Build history of the part. All positions in model axes, mm. Round coordinates to 2 decimals unless told otherwise and drop trailing zeros. Write each loop counter-clockwise with the first axis right and the second up, starting at its lowest first coordinate (ties: lowest second). Pieces come first, ordered by that corner, then holes. Notation, with made-up numbers: (-18, 64) - (-13, 64) arc R14 ccw to (-13, 81) - close; hole circle Ø2 at (69, 71). An arc over 180 degrees is marked (long way). Write each question's results on one line, items separated by ' | '.
Autodesk Inventor part; units mm, degrees
ref_plane "Work Plane1" through (-4668.2945, 0, 0) normal (0, 0, 1) x (1, 0, 0)
ref_plane "YZ Plane" through (0, 0, 0) normal (1, 0, 0) x (0, 1, 0)
ref_plane "XZ Plane" through (0, 0, 0) normal (0, 1, 0) x (-1, 0, 0)
ref_plane "Work Plane1" through (-4668.2945, 0, 0) normal (0, 0, 1) x (1, 0, 0)
sketch "Sketch1" plane through (-4668.2945, 0, 0) normal (0, 0, 1) x (1, 0, 0)
  line L0 (0, 19.05) -> (466.725, 19.05)
  line L1 (466.725, 0) -> (466.725, 19.05)
  line L2 (0, 0) -> (0, 19.05)
  line L3 (0, -340.481) -> (0, -321.431)
  line L4 (466.725, -340.481) -> (0, -340.481)
  line L5 (466.725, -340.481) -> (0, -340.481)
  line L6 (466.725, -340.481) -> (466.725, -321.431)
  line L7 (0, -321.431) -> (466.725, -321.431) construction
  line L8 (0, -340.481) -> (0, -321.431)
  line L9 (466.725, 19.05) -> (0, 19.05)
  line L10 (0, 19.05) -> (0, -340.481) construction
  line L11 (466.725, -340.481) -> (466.725, 19.05) construction
  line L12 (147.3639, -408.7465) -> (46.3111, -408.7465) construction
  line L13 (466.725, -340.481) -> (466.725, -408.7465) construction
  line L14 (466.725, -408.7465) -> (147.3639, -408.7465) construction
  line L15 (46.3111, -408.7465) -> (0, -408.7465)
  line L16 (0, -408.7465) -> (0, -340.481) construction
  line L17 (466.725, -408.7465) -> (466.725, -434.1465)
  line L18 (466.725, -434.1465) -> (0, -434.1465)
  line L19 (0, -434.1465) -> (0, -408.7465)
  line L20 (400.05, 19.05) -> (400.05, 0)
  line L21 (400.05, -321.431) -> (400.05, -340.481)
  line L22 (400.05, 0) -> (400.05, -321.431)
  line L23 (400.05, -340.481) -> (400.05, -434.1465)
  line L24 (101.6, 19.05) -> (101.6, 0)
  line L25 (101.6, -321.431) -> (101.6, -340.481)
  line L26 (101.6, 0) -> (101.6, -321.431)
  line L27 (101.6, -340.481) -> (101.6, -434.1465)
  point P0 (4668.2945, 0)
  point P1 (50.8, 19.05)
  point P2 (50.8, -321.431)
  point P3 (50.8, -340.481)
  point P4 (50.8, -434.1465)
  dimension "d7" = 25.4
extrude "Extrusion1" add sketch "Sketch1" along normal blind 19.05
sketch "Sketch2" plane through (-4668.2945, 0, 0) normal (0, 0, -1) x (-1, 0, 0)
  line L0 (-232.5687, -355.978) -> (-232.5688, 34.547)
  line L1 (-141.2875, -408.7465) -> (-141.2875, 124.6535)
  circle A0 centre (-186.9249, -370.6465) radius 15.875
  line L2 (-232.5687, -370.6465) -> (-141.2875, -370.6465) construction
  line L3 (0, -408.7465) -> (-466.725, -408.7465)
  point P0 (-4668.2945, 0)
  dimension "d2" = 31.75
  dimension "d3" = 45.6438
  dimension "d4" = 38.1
extrude "Extrusion2" cut sketch "Sketch2" against normal up to next
sketch "Sketch3" plane through (-4668.2945, 0, 0) normal (0, 0, -1) x (-1, 0, 0)
  circle A0 centre (-186.9249, -370.6465) radius 15.875
  arc A1 (-207.9625, -430.5603) -> (-155.5881, -425.8756) centre (-186.9249, -370.6465) ccw
  line L0 (-101.6, -434.1465) -> (-400.05, -434.1465)
  line L1 (0, -340.481) -> (-157.1625, -426.7397)
  line L2 (-466.725, -340.481) -> (-207.9625, -430.5603)
  line L3 (-466.725, -434.1465) -> (-466.725, -340.481)
  line L4 (-466.725, -434.1465) -> (-466.725, 19.05)
  line L5 (-101.6, -434.1465) -> (-400.05, -434.1465)
  line L6 (0, -434.1465) -> (0, -340.481)
  line L7 (0, 19.05) -> (0, -434.1465)
  arc A2 (-155.5881, -425.8756) -> (-207.9625, -430.5603) centre (-186.9249, -370.6465) ccw construction
  line L8 (-101.6, 19.05) -> (-101.6, -434.1465)
  line L9 (-101.6, -396.2442) -> (-101.6, -434.1465)
  line L10 (-400.05, -434.1465) -> (-400.05, 19.05)
  line L11 (-400.05, -363.6916) -> (-400.05, -434.1465)
  point P0 (-4668.2945, 0)
  point P1 (-186.9249, -434.1465)
  point P2 (-50.8, -434.1465)
extrude "Extrusion3" cut sketch "Sketch3" against normal blind 19.05
sketch "Sketch4" plane through (-4668.2945, 0, 19.05) normal (0, 0, 1) x (1, 0, 0)
  circle A0 centre (316.7063, -160.7155) radius 12.7 construction
  circle A1 centre (316.7063, -160.7155) radius 50.8
  point P0 (4668.2945, 0)
  dimension "d10" = 101.6
extrude "Extrusion4" cut sketch "Sketch4" against normal up to next
properties part number "cannonSideWall"
(1) Slice it at A-A, the plane y = -155.5. Write the cut outline in (x, z).
Worked answers:
outline: (-4566.69, 0) - (-4402.12, 0) - (-4402.12, 19.05) - (-4566.69, 19.05) - close; (-4301.06, 0) - (-4268.24, 0) - (-4268.24, 19.05) - (-4301.06, 19.05) - close
(2) Slice it at B-B, the plane x = -4356.5. Write the cut outline in (y, z), and give its area (3 significant figures).
Worked answers:
outline: (-394.41, 0) - (-211.28, 0) - (-211.28, 19.05) - (-394.41, 19.05) - close; (-110.15, 0) - (19.05, 0) - (19.05, 19.05) - (-110.15, 19.05) - close | area: 5,950 mm2
(3) Slice it at C-C, the plane z = 5.5. State how many separate pieces and enclosed holes the cut face has, and give its area (3 significant figures).
Worked answers:
separate pieces: 1 | enclosed holes: 2 | area: 118,000 mm2
(4) Drill centre lines: probe 1 along X at (y, z) = (-129, 9.75); probe 2 along Y at (x, z) = (-4306.5, 9.75); probe 3 along Y at (x, z) = (-4364, 9.5). Where is each one in solid material? Low to high. Write a range as [from, to].
Worked answers:
probe 1: x = [-4566.69, -4391.27], [-4311.9, -4268.24] | probe 2: y = [-377.01, -184.12], [-137.31, 19.05] | probe 3: y = [-397.03, -209.98], [-111.46, 19.05]
(5) Flat gauge pins, fed straight in: pin 1 Ø4 at (x, z) = (-4504, 12.5) entering from -Y; pin 2 Ø1 at (x, z) = (-4408, 13.5) entering from -Y; pin 3 Ø5 at (x, z) = (-4418, 11.5) entering from -Y. Where does each tip first touch, or does it go through?
Worked answers:
pin 1: stops at y = -430.7 | pin 2: stops at y = -412.52 | pin 3: stops at y = -416.69
(6) Slice it at D-D, the plane x = -4445. Write the cut outline in (y, z).
Worked answers:
outline: (-425.22, 0) - (19.05, 0) - (19.05, 19.05) - (-425.22, 19.05) - close
(7) Two-plate mould, pull along X, no slides. Class faces 1 (the flat face through (-4268.244, -170, 9)), 2 (the cylindrical face through (-4465.51, -369.95, 9.39)), 3 (the flat face through (-4420, -204, 0)): released by +X, released by -X, zero draft, split by the parting line, or undercut.
Worked answers:
face 1: released by +X | face 2: undercut | face 3: zero draft
